```python
from build123d import *

# Parameters (mm, degrees)
F0_R     = 12.5
F1_DEPTH = 8
F2_R     = 7
F3_DEPTH = 5
F4_R     = 5
F5_DEPTH = 25
F6_R     = 9
F7_DEPTH = 4
F8_R     = 2


with BuildPart() as f1:
    # F0 (on Top) → F1 (new body)
    with BuildSketch(Plane.XY):
        Circle(F0_R)
    extrude(amount=F1_DEPTH)

    # F2 (on face) → F3 (join)
    with BuildSketch(Plane.XY.offset(8)):
        Circle(F2_R)
    extrude(amount=F3_DEPTH)

    # F4 (on face) → F5 (cut)
    with BuildSketch(Plane.XY.offset(13)):
        Circle(F4_R)
    extrude(amount=-F5_DEPTH, mode=Mode.SUBTRACT)

    # F6 (on face) → F7 (cut)
    with BuildSketch(Plane(origin=(0, 0, 0), x_dir=(1, 0, 0), z_dir=(0, 0, -1))):
        Circle(F6_R)
    extrude(amount=-F7_DEPTH, mode=Mode.SUBTRACT)

    # F8
    f8_edges = [f1.edges().sort_by_distance(p)[0] for p in [
        (-12.5, 0, 0),
        (-12.5, 0, 8),
    ]]
    fillet(f8_edges, radius=F8_R)


solid = f1.part
```
Design review of the part built by this model. Coordinates are the model's own, in mm. A direction names the side the tool comes from. Coordinates: 2 decimals unless noted, no trailing zeros. Order: outer loops, then holes, each group sorted by start corner. A loop starts at its lowest first (then second) coordinate and runs counter-clockwise, first axis right, second up. Notation, with made-up numbers: (13.5, 71) - (58.5, 71) arc R7 cw to (58.5, 79) - close; hole circle Ø7 at (-38.5, -14.75). An arc over 180 degrees is marked (long way). Answer in a Markdown table with one row per item.
(1) Wall thickness on line 1 along Y through (x, z) = (0, 1.9); line 2 along Y through (x, z) = (0, 10.75); line 3 along X through (y, z) = (-0.25, 4.5): over which ranges is each line inside the solid? List them lowest first. Write a range as from..to.
Checked values:
| item | result |
|---|---|
| line 1 | -12.5..-9, 9..12.5 |
| line 2 | -7..-5, 5..7 |
| line 3 | -12.5..-4.99, 4.99..12.5 |
(2) Consider section C-C on z = 4.75. State the section outline as (x, y) points, plus the area to 3 significant figures.
Checked values:
| item | result |
|---|---|
| outline | circle Ø25 at (0, 0); hole circle Ø10 at (0, 0) |
| area | 412 mm^2 |
(3) Clearance check with flat-ended pins moving along their axes: pin 1 (1 mm diameter, centred on x = -5.5, z = 2, fed in from +Y); pin 2 (1.5 mm diameter, centred on x = 5, z = 8.5, fed in from -Y); pin 3 (2 mm diameter, centred on y = -9.5, z = 4, fed in from -X); pin 4 (1 mm diameter, centred on x = 3, y = -0.5, fed in from -Z). State where each tip first meets the part, or that it passes through.
Checked values:
| item | result |
|---|---|
| pin 1 | y = 11.46 |
| pin 2 | y = -10.36 |
| pin 3 | x = -9.17 |
| pin 4 | through |
(4) Consider section A-A on y = 0. State the section outline as (x, z) points.
Checked values:
| item | result |
|---|---|
| outline | (-12.5, 2) arc R2 ccw to (-10.5, 0) - (-9, 0) - (-9, 4) - (-5, 4) - (-5, 13) - (-7, 13) - (-7, 8) - (-10.5, 8) arc R2 ccw to (-12.5, 6) - close; (5, 4) - (9, 4) - (9, 0) - (10.5, 0) arc R2 ccw to (12.5, 2) - (12.5, 6) arc R2 ccw to (10.5, 8) - (7, 8) - (7, 13) - (5, 13) - close |
(5) The part is to be moulded in two halves that separate along X. For faces 3 (the flat face through (2, -7, 8)), 4 (the flat face through (4, 4, 4)), 5 (the cylindrical face through (-1.08, -4.88, 8.56)), 6 (the cylindrical face through (6.466, -2.681, 10.465)), say which applies: released by +X, released by -X, zero draft, split by the parting line, or undercut.
Checked values:
| item | result |
|---|---|
| face 3 | zero draft |
| face 4 | undercut |
| face 5 | undercut |
| face 6 | split by the parting line |
(6) For faces 1 (the cylindrical face through (-1.172, -8.923, 1.972)), 2 (the flat face through (-2, 5, 13)), list the 3-axis set-ups (+Z, -Z, +X, -X, +Y, -Y) from which the entire face can be reached by the end or side of a thin tool; tool diameter is ignored.
Checked values:
| item | result |
|---|---|
| face 1 | -Z |
| face 2 | +Z, +X, -X, +Y, -Y |
